For this review, use the dimensioned drawing (mm, ordinates from the lowest corner) and the shaded views. Round coordinates to 2 decimals unless told otherwise and drop trailing zeros. Write each loop counter-clockwise with the first axis right and the second up, starting at its lowest first coordinate (ties: lowest second). Pieces come first, ordered by that corner, then holes. Notation, with made-up numbers: (88.5, 74) - (95.5, 74) arc R34 cw to (95.5, 110) - close; hole circle Ø9 at (88, 5). An arc over 180 degrees is marked (long way). Return JSON: item names as keys, results as strings.
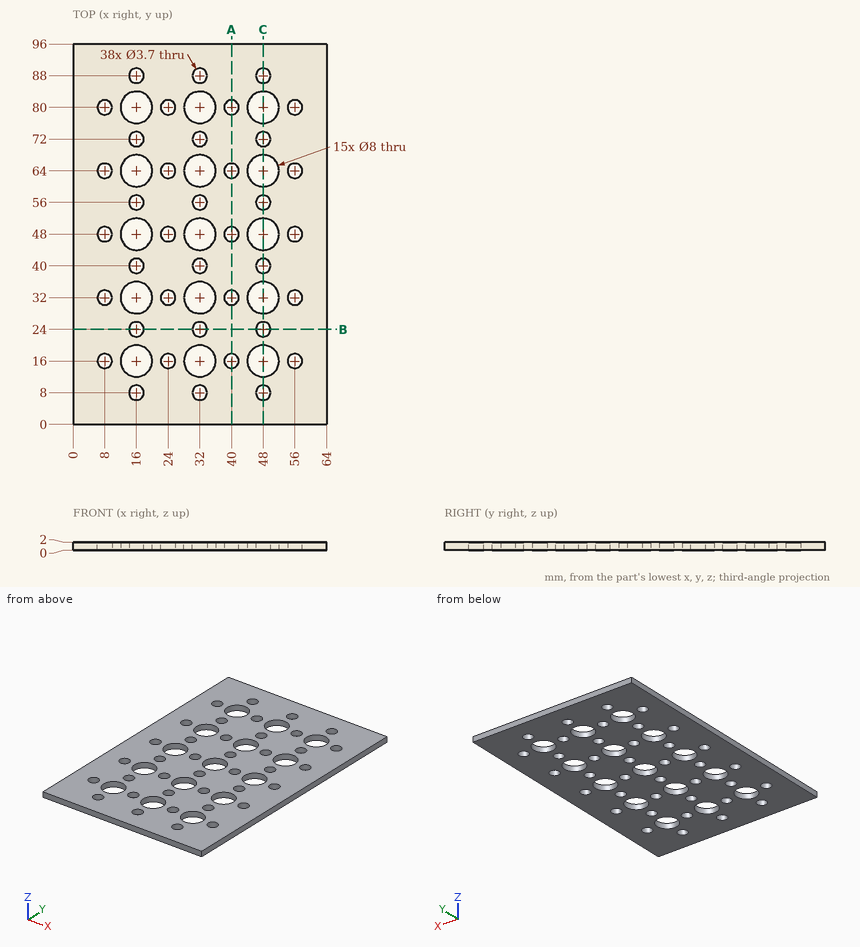
(1) Add section C-C (x = 48). Give the number of separate pieces and of enclosed holes in the cut face, plus the area to 3 significant figures.
Filled in:
{"separate pieces": "12", "enclosed holes": "0", "area": "67.6 mm2"}
(2) Wall thickness on line 1 (Y direction, x = 40, z = 1); line 2 (X direction, y = 88, z = 1.05); line 3 (X direction, y = 51, z = 1.2): over which ranges is each line inside the solid? List them lowest first.
Filled in:
{"line 1": "y = 0 to 14.15, 17.85 to 30.15, 33.85 to 46.15, 49.85 to 62.15, 65.85 to 78.15, 81.85 to 96", "line 2": "x = 0 to 14.15, 17.85 to 30.15, 33.85 to 46.15, 49.85 to 64", "line 3": "x = 0 to 13.35, 18.65 to 29.35, 34.65 to 45.35, 50.65 to 64"}
(3) Add section B-B (y = 24). Write out the cut boundary in (x, z).
Filled in:
{"outline": "(0, 0) - (14.15, 0) - (14.15, 2) - (0, 2) - close; (17.85, 0) - (30.15, 0) - (30.15, 2) - (17.85, 2) - close; (33.85, 0) - (46.15, 0) - (46.15, 2) - (33.85, 2) - close; (49.85, 0) - (64, 0) - (64, 2) - (49.85, 2) - close"}
(4) Add section A-A (x = 40). Write out the cut boundary in (y, z).
Filled in:
{"outline": "(0, 0) - (14.15, 0) - (14.15, 2) - (0, 2) - close; (17.85, 0) - (30.15, 0) - (30.15, 2) - (17.85, 2) - close; (33.85, 0) - (46.15, 0) - (46.15, 2) - (33.85, 2) - close; (49.85, 0) - (62.15, 0) - (62.15, 2) - (49.85, 2) - close; (65.85, 0) - (78.15, 0) - (78.15, 2) - (65.85, 2) - close; (81.85, 0) - (96, 0) - (96, 2) - (81.85, 2) - close"}
